from build123d import *

# Parameters (mm, degrees)
PAD_DEPTH       = 60
POCKET_DEPTH    = 50
POCKET001_DEPTH = 407.8842315097
POCKET002_DEPTH = 407.6818719776
SKETCH004_W     = 462.917107
SKETCH004_H     = 152.532247
SKETCH004_W_2   = 206.430237
SKETCH004_H_2   = 142.147327
POCKET003_DEPTH = 60.001
SKETCH005_R     = 2.05
SKETCH005_W     = 1
SKETCH005_H     = 40
POCKET004_DEPTH = 10.001


with BuildPart() as part:
    # Sketch → Pad (new body)
    with BuildSketch(Plane.XY):
        Polygon((450, 0), (450, 90), (356, 88.12), (355.76, 100.12), (343.76, 99.88), (344, 87.88), (6, 81.12), (5.76, 93.12), (-6.24, 92.88), (-6, 80.88), (-50, 80), (-50, 0), align=None)
    extrude(amount=PAD_DEPTH)

    # Sketch001 (on Face14 of Pad) → Pocket (cut)
    with BuildSketch(Plane.XY.offset(60)):
        Polygon((-50, 10), (-50, 79), (450, 79), (450, 0), (356, 1.88), (356.2, 11.88), (344.2, 12.12), (344, 2.12), (6, 8.88), (6.2, 18.88), (-5.8, 19.12), (-6, 9.12), align=None)
    extrude(amount=-POCKET_DEPTH, mode=Mode.SUBTRACT)

    # Sketch002 (on Face26 of Pocket) → Pocket001 (cut, through all)
    with BuildSketch(Plane(origin=(355.8200719712, -7.1164014394, 0), x_dir=(0.0199960012, 0.99980006, 0), z_dir=(0.99980006, -0.0199960012, 0))):
        with BuildLine():
            ThreePointArc((19.0002003399, 54), (15.5006314384, 55.4495689014), (16.9502003399, 51.95))
            ThreePointArc((16.9502003399, 51.95), (13.3347157657, 39), (16.9502003399, 26.05))
            ThreePointArc((16.9502003399, 26.05), (15.5006314384, 22.5504310986), (19.0002003399, 24))
            Line((19.0002003399, 24), (19.0002003399, 54))
        make_face()
    extrude(amount=-POCKET001_DEPTH, mode=Mode.SUBTRACT)

    # Sketch003 (on Face14 of Pocket001) → Pocket002 (cut, through all)
    with BuildSketch(Plane(origin=(357.6193522591, 7.1523870452, 0), x_dir=(-0.0199960012, 0.99980006, 0), z_dir=(0.99980006, 0.0199960012, 0))):
        with BuildLine():
            ThreePointArc((92.9862046184, 54), (89.486635717, 55.4495689014), (90.9362046184, 51.95))
            ThreePointArc((90.9362046184, 51.95), (87.3207200443, 39), (90.9362046184, 26.05))
            ThreePointArc((90.9362046184, 26.05), (89.486635717, 22.5504310986), (92.9862046184, 24))
            Line((92.9862046184, 24), (92.9862046184, 54))
        make_face()
    extrude(amount=-POCKET002_DEPTH, mode=Mode.SUBTRACT)

    # Sketch004 (on Face7 of Pocket002) → Pocket003 (cut, through all)
    with BuildSketch(Plane.XY.offset(60)):
        with Locations((113.5414465, 49.6986895)):
            Rectangle(SKETCH004_W, SKETCH004_H)
        with Locations((458.2151185, 57.1989195)):
            Rectangle(SKETCH004_W_2, SKETCH004_H_2)
    extrude(amount=-POCKET003_DEPTH, mode=Mode.SUBTRACT)

    # Sketch005 (on Face2 of Pocket003) → Pocket004 (cut, through all)
    with BuildSketch(Plane(origin=(345, 0, 0), x_dir=(0, -1, 0), z_dir=(-1, 0, 0))):
        with Locations((-86, 8)):
            Circle(SKETCH005_R)
        with Locations((-0.5, 30)):
            Rectangle(SKETCH005_W, SKETCH005_H)
        Polygon((-87.9048, 60), (-79, 60), (-79, 10), (-87.9048, 18.95854), align=None)
    extrude(amount=-POCKET004_DEPTH, mode=Mode.SUBTRACT)


solid = part.part
Model file for the job. Use its own axes, mm. A direction names the side the tool comes from. Give positions to 0.01 mm unless a question says otherwise; leave off trailing zeros. Order: outer loops, then holes, each group sorted by start corner. A loop starts at its lowest first (then second) coordinate and runs counter-clockwise, first axis right, second up. Notation, with made-up numbers: (76, 6) -> (105, 6) arc R18 ccw to (105, 22) -> close; hole circle Ø1 at (-3.75, 18). An arc over 180 degrees is marked (long way). Use CSV: the item, a comma, the result in double quotes.
1. Mould opens along Z. For faces 6 (the flat face through (350, 51, 0)), 7 (the flat face through (350, 1, 30)), 8 (the flat face through (350, 0, 55)), 9 (the flat face through (350, 94, 60)) say: +Z half, -Z half, draft (parallel to the pull), parting line (faces both ways), or undercut.
Outcome:
face 6,"-Z half"
face 7,"undercut"
face 8,"draft"
face 9,"+Z half"
2. Drill centre lines: line 1 along Z through (x, y) = (347.75, 86); line 2 along Z through (x, y) = (350, 68.5); line 3 along Y through (x, z) = (351.5, 21). Where is each one in solid material? Low to high. Write a range as from..to.
Outcome:
line 1,"0..5.95, 10.05..17.04"
line 2,"0..10"
line 3,"1..11.97, 87.9..100.03"
3. Drop flat-ended pins along their axis: pin 1 (5 mm diameter, centred on x = 348, y = 58, fed in from +Z); pin 2 (1.5 mm diameter, centred on x = 347, z = 36, fed in from -Y). Give the stop position or say it passes through.
Outcome:
pin 1,"z = 10"
pin 2,"y = 1"
4. Band-saw the part on B-B, the plane y = 86. Give the cut face in (x, z), then the cut area to 3 significant figures.
Outcome:
outline,"(345, 0) -> (355, 0) -> (355, 5.95) -> (345, 5.95) -> close; (345, 10.05) -> (355, 10.05) -> (355, 17.04) -> (345, 17.04) -> close"
area,"129 mm²"
5. Band-saw the part on C-C, the plane y = 14. Give the cut face in (x, z), then the cut area to 3 significant figures.
Outcome:
outline,"(345, 0) -> (355, 0) -> (355, 10) -> (345, 10) -> close"
area,"100 mm²"
6. 3-axis set-ups, long thin cutter, end or side, ignore diameter. For faces 1 (the cylindrical face through (350.1, 94.34, 39.19)), 2 (the cylindrical face through (350.1, 96.56, 55.5)), 3 (the flat face through (350, 0, 5)), 4 (the flat face through (355, 50, 8)), 5 (the flat face through (349.93, 83.39, 14.417)): which of +Z, -Z, +X, -X, +Y, -Y reach the whole face in a straight line?
Outcome:
face 1,"-X, +Y"
face 2,"none"
face 3,"+Z, -Z, +X, -X, -Y"
face 4,"+Z, -Z, +X, +Y, -Y"
face 5,"+Z, +X, -X"
7. Band-saw the part on A-A, the plane z = 8. Give the cut face in (x, y), then the cut area to 3 significant figures.
Outcome:
outline,"(345, 0) -> (355, 0) -> (355, 83.95) -> (345, 83.95) -> close; (345, 88.05) -> (355, 88.05) -> (355, 100.1) -> (345, 99.9) -> close"
area,"959 mm²"
